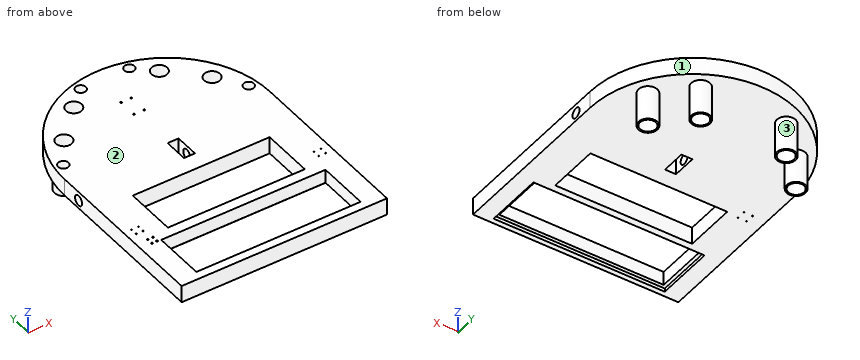
```python
from build123d import *

# Parameters (mm, degrees)
SKETCH_1_R           = 23
EXTRUDE_1_DEPTH      = 50
EXTRUDE_START        = 100
SKETCH_2_R           = 27.5
SKETCH_2_R_2         = 23
EXTRUDE_2_DEPTH      = 100
SKETCH_3_R           = 15
CUT_EXTRUDE_1_DEPTH  = 788.400787401
SKETCH_4_W           = 32
SKETCH_4_H           = 70
CUT_EXTRUDE_2_DEPTH  = 100
SKETCH_5_W           = 400
SKETCH_5_H           = 150
CUT_EXTRUDE_3_DEPTH  = 603.07972894
SKETCH_6_W           = 480
SKETCH_6_H           = 150
CUT_EXTRUDE_4_DEPTH  = 100
SKETCH_7_W           = 500
SKETCH_7_H           = 170
CUT_EXTRUDE_5_DEPTH  = 10
SKETCH_9_R           = 2.25
CUT_EXTRUDE_6_DEPTH  = 5
SKETCH_10_R          = 15
CUT_EXTRUDE_7_DEPTH  = 30
SKETCH_11_R          = 2.25
CUT_EXTRUDE_8_DEPTH  = 30
SKETCH_12_R          = 1.5
CUT_EXTRUDE_9_DEPTH  = 10
SKETCH_13_R          = 1.5
CUT_EXTRUDE_10_DEPTH = 10


with BuildPart() as part:
    # 草图1 → 凸台-拉伸1 (new body)
    with BuildSketch(Plane.XY):
        with BuildLine():
            Line((-300, 0), (-300, -500))
            Line((-300, -500), (300, -500))
            Line((300, -500), (300, 0))
            ThreePointArc((300, 0), (0, 300), (-300, 0))
        make_face()
        with Locations((-216.506350946, 125)):
            Circle(SKETCH_1_R, mode=Mode.SUBTRACT)
        with Locations((-125, 216.506350946)):
            Circle(SKETCH_1_R, mode=Mode.SUBTRACT)
        with Locations(Location((125, 216.506350946, 0), (0, 0, 180))):
            Circle(SKETCH_1_R, mode=Mode.SUBTRACT)
        with Locations(Location((216.506350946, 125, 0), (0, 0, 180))):
            Circle(SKETCH_1_R, mode=Mode.SUBTRACT)
    extrude(amount=EXTRUDE_1_DEPTH)

    # 草图2 → 凸台-拉伸2 (add)
    # profile 1 of 4: a face of its own
    with BuildSketch(Plane(origin=(0, 0, 0), x_dir=(-1, 0, 0), z_dir=(0, 0, -1)).offset(EXTRUDE_START)):
        with Locations(Location((-216.506350946, 125, 0), (0, 0, 180))):
            Circle(SKETCH_2_R)
        with Locations((-216.506350946, 125)):
            Circle(SKETCH_2_R_2, mode=Mode.SUBTRACT)
    # profile 2 of 4: a face of its own
    with BuildSketch(Plane(origin=(0, 0, 0), x_dir=(-1, 0, 0), z_dir=(0, 0, -1)).offset(EXTRUDE_START)):
        with Locations(Location((-125, 216.506350946, 0), (0, 0, 180))):
            Circle(SKETCH_2_R)
        with Locations((-125, 216.506350946)):
            Circle(SKETCH_2_R_2, mode=Mode.SUBTRACT)
    # profile 3 of 4: a face of its own
    with BuildSketch(Plane(origin=(0, 0, 0), x_dir=(-1, 0, 0), z_dir=(0, 0, -1)).offset(EXTRUDE_START)):
        with Locations(Location((216.506350946, 125, 0), (0, 0, 180))):
            Circle(SKETCH_2_R)
        with Locations(Location((216.506350946, 125, 0), (0, 0, 180))):
            Circle(SKETCH_2_R_2, mode=Mode.SUBTRACT)
    # profile 4 of 4: a face of its own
    with BuildSketch(Plane(origin=(0, 0, 0), x_dir=(-1, 0, 0), z_dir=(0, 0, -1)).offset(EXTRUDE_START)):
        with Locations(Location((125, 216.506350946, 0), (0, 0, 180))):
            Circle(SKETCH_2_R)
        with Locations(Location((125, 216.506350946, 0), (0, 0, 180))):
            Circle(SKETCH_2_R_2, mode=Mode.SUBTRACT)
    extrude(amount=-EXTRUDE_2_DEPTH)

    # 草图3 → 切除-拉伸1 (cut, through all)
    with BuildSketch(Plane.ZY.offset(300)):
        with Locations((23.548349361, -60)):
            Circle(SKETCH_3_R)
    extrude(amount=-CUT_EXTRUDE_1_DEPTH, mode=Mode.SUBTRACT)

    # 草图4 → 切除-拉伸2 (cut)
    with BuildSketch(Plane.XY.offset(50)):
        with Locations((0, -60)):
            Rectangle(SKETCH_4_W, SKETCH_4_H)
    extrude(amount=-CUT_EXTRUDE_2_DEPTH, mode=Mode.SUBTRACT)

    # 草图5 → 切除-拉伸3 (cut, through all)
    with BuildSketch(Plane.XY.offset(50)):
        with Locations((0, -220)):
            Rectangle(SKETCH_5_W, SKETCH_5_H)
    extrude(amount=-CUT_EXTRUDE_3_DEPTH, mode=Mode.SUBTRACT)

    # 草图6 → 切除-拉伸4 (cut)
    with BuildSketch(Plane.XY.offset(50)):
        with Locations((0, -400)):
            Rectangle(SKETCH_6_W, SKETCH_6_H)
    extrude(amount=-CUT_EXTRUDE_4_DEPTH, mode=Mode.SUBTRACT)

    # 草图7 → 切除-拉伸5 (cut)
    with BuildSketch(Plane(origin=(0, 0, 0), x_dir=(-1, 0, 0), z_dir=(0, 0, -1))):
        with Locations((0, -400)):
            Rectangle(SKETCH_7_W, SKETCH_7_H)
    extrude(amount=-CUT_EXTRUDE_5_DEPTH, mode=Mode.SUBTRACT)

    # 草图9 → 切除-拉伸6 (cut)
    with BuildSketch(Plane.XY.offset(50)):
        with Locations((10, 113.043497002)):
            Circle(SKETCH_9_R)
        with Locations((-20, 113.043497002)):
            Circle(SKETCH_9_R)
        with Locations((-20, 168.205707409)):
            Circle(SKETCH_9_R)
        with Locations((10, 168.205707409)):
            Circle(SKETCH_9_R)
    extrude(amount=-CUT_EXTRUDE_6_DEPTH, mode=Mode.SUBTRACT)

    # 草图10 → 切除-拉伸7 (cut)
    with BuildSketch(Plane.XY.offset(50)):
        with Locations((-270.822132078, 47.753248858)):
            Circle(SKETCH_10_R)
        with Locations((-71.175237403, 265.629602229)):
            Circle(SKETCH_10_R)
        with Locations(Location((270.822132078, 47.753248858, 0), (0, 0, 180))):
            Circle(SKETCH_10_R)
        with Locations(Location((71.175237403, 265.629602229, 0), (0, 0, 180))):
            Circle(SKETCH_10_R)
    extrude(amount=-CUT_EXTRUDE_7_DEPTH, mode=Mode.SUBTRACT)

    # 草图11 → 切除-拉伸8 (cut)
    with BuildSketch(Plane.XY.offset(50)):
        with Locations((-265.77797753, -305.157271427)):
            Circle(SKETCH_11_R)
        with Locations((-250.77797753, -305.157271427)):
            Circle(SKETCH_11_R)
        with Locations((-265.77797753, -322.957271427)):
            Circle(SKETCH_11_R)
        with Locations((-250.77797753, -322.957271427)):
            Circle(SKETCH_11_R)
    extrude(amount=-CUT_EXTRUDE_8_DEPTH, mode=Mode.SUBTRACT)

    # 草图12 → 切除-拉伸9 (cut)
    with BuildSketch(Plane.XY.offset(50)):
        with Locations((-276.542958653, -251.964088139)):
            Circle(SKETCH_12_R)
        with Locations((-256.542958653, -251.964088139)):
            Circle(SKETCH_12_R)
        with Locations((-276.542958653, -271.964088139)):
            Circle(SKETCH_12_R)
        with Locations((-256.542958653, -271.964088139)):
            Circle(SKETCH_12_R)
    cut_extrude_9 = extrude(amount=-CUT_EXTRUDE_9_DEPTH, mode=Mode.SUBTRACT)

    # 镜向1: 切除-拉伸9 across plane
    add(cut_extrude_9.mirror(Plane(origin=(0, 0, 0), x_dir=(0, 0, 1), z_dir=(1, 0, 0))), mode=Mode.SUBTRACT)

    # 草图13 → 切除-拉伸10 (cut)
    with BuildSketch(Plane(origin=(0, 0, 0), x_dir=(-1, 0, 0), z_dir=(0, 0, -1))):
        with Locations((259.167415515, -123.923585862)):
            Circle(SKETCH_13_R)
        with Locations((234.167415515, -123.923585862)):
            Circle(SKETCH_13_R)
        with Locations((234.167415515, -148.923585862)):
            Circle(SKETCH_13_R)
        with Locations((259.167415515, -148.923585862)):
            Circle(SKETCH_13_R)
    extrude(amount=-CUT_EXTRUDE_10_DEPTH, mode=Mode.SUBTRACT)


solid = part.part
```
Input: part model. Units: mm. Frame: model coordinates. Face numbers are marked on the shaded views. Coordinates: 2 decimals unless noted, no trailing zeros. Loops run counter-clockwise (first coordinate to the right, second up) from the corner with the lowest first, then second, coordinate; pieces in that order, holes last.
Q1. Section B-B, the plane x = -74.5. Return the cut outline in (y, z), and give its area (3 significant figures).
Results are:
outline: (-500, 0) - (-485, 0) - (-485, 10) - (-475, 10) - (-475, 50) - (-500, 50) - close; (-325, 10) - (-315, 10) - (-315, 0) - (-295, 0) - (-295, 50) - (-325, 50) - close; (-145, 0) - (290.6, 0) - (290.6, 50) - (280.26, 50) - (280.26, 20) - (251, 20) - (251, 50) - (-145, 50) - close; hole circle Ø30 at (-60, 23.55)
area: 22,700 mm2
Q2. Line query: line 1 along X through (y, z) = (125, -65); line 2 along Y through (x, z) = (10, 47); line 3 along X through (y, z) = (215.5, 18). Output: solid intervals per line, ascending.
Results are:
line 1: x = -244.01 to -239.51, -193.51 to -189.01, 189.01 to 193.51, 239.51 to 244.01
line 2: y = -500 to -475, -325 to -295, -145 to -95, -25 to 110.79, 115.29 to 165.96, 170.46 to 299.83
line 3: x = -208.71 to -147.98, -102.02 to 102.02, 147.98 to 208.71
Q3. Section D-D, the plane y = 125. Return the cut outline in (x, z).
Results are:
outline: (-272.72, 0) - (-244.01, 0) - (-244.01, -100) - (-239.51, -100) - (-239.51, 50) - (-272.72, 50) - close; (-193.51, -100) - (-189.01, -100) - (-189.01, 0) - (189.01, 0) - (189.01, -100) - (193.51, -100) - (193.51, 50) - (-193.51, 50) - close; (239.51, -100) - (244.01, -100) - (244.01, 0) - (272.72, 0) - (272.72, 50) - (239.51, 50) - close
Q4. Contact query for flat-ended pins moving along their axis: pin 1 (2.5 mm diameter, centred on x = -259.17, y = -148.92, fed in from -Z); pin 2 (20 mm diameter, centred on x = 53.5, z = 36, fed in from +Y); pin 3 (15 mm diameter, centred on x = -264.5, y = 51.5, fed in from +Z); pin 4 (1 mm diameter, centred on x = -52, y = -293.5, fed in from -Z). Output: stop coordinate, or through.
Results are:
pin 1: stops at z = 10
pin 2: stops at y = 296.83
pin 3: stops at z = 20
pin 4: passes through
Q5. Section C-C, the plane y = -60. Return the cut outline in (x, z).
Results are:
outline: (-300, 0) - (-16, 0) - (-16, 8.55) - (-300, 8.55) - close; (-300, 38.55) - (-16, 38.55) - (-16, 50) - (-300, 50) - close; (16, 0) - (300, 0) - (300, 8.55) - (16, 8.55) - close; (16, 38.55) - (300, 38.55) - (300, 50) - (16, 50) - close
Q6. Section A-A, the plane z = -57. Return the cut outline in (x, y).
Results are:
outline: circle Ø55 at (-216.51, 125); circle Ø55 at (-125, 216.51); circle Ø55 at (125, 216.51); circle Ø55 at (216.51, 125); hole circle Ø46 at (-216.51, 125); hole circle Ø46 at (-125, 216.51); hole circle Ø46 at (125, 216.51); hole circle Ø46 at (216.51, 125)
Q7. Mould query, pull axis X, two halves, no side actions, for the marked faces 1, 2 and 3. Classes: +X half, -X half, draft (parallel to the pull), parting line (faces both ways), or undercut.
Results are:
face 1: parting line
face 2: draft
face 3: undercut
